Geometry check sheet. Reference: the model listing, model coordinates, mm. A direction names the side the tool comes from. Coordinates: 2 decimals unless noted, no trailing zeros. Write each loop counter-clockwise with the first axis right and the second up, starting at its lowest first coordinate (ties: lowest second). Pieces come first, ordered by that corner, then holes. Notation, with made-up numbers: (0.25, -7.75) -> (17.25, -7.75) arc R20 ccw to (17.25, 0.25) -> close; hole circle Ø11 at (-21, 83.5). An arc over 180 degrees is marked (long way). Answer in a Markdown table with one row per item. Add a question column.
1. Cross-section at B-B on z = 0. Record the cut outline in (x, y), and give its area (3 significant figures).
2. Cross-section at C-C on y = 182.5. Record the cut outline in (x, z).
3. Cross-section at A-A on x = 0. Record the cut outline in (y, z), and give its area (3 significant figures).
4. Set-up check for faces 4 (the cylindrical face through (3.69, 202.9, 51.92)), 5 (the flat face through (98.3, 20, 18.3)), 6 (the conical face through (-12.65, 102.63, -56.98)): record each of +Z, -Z, +X, -X, +Y, -Y from which the full face is reachable in a straight line by a thin tool's end or side.
5. Depth check by flat-ended pin: P1, Ø3, axis at x = -41.5, z = 73.5, coming from the -Y side; P2, Ø8, axis at y = 215, z = -56.5, coming from the +X side; P3, Ø12, axis at x = 25.5, z = -26, coming from the +Y side; P4, Ø12, axis at y = 36, z = 10, coming from the -X side. Enter the tip coordinate at first touch or a pass-through.
6. Scan lines: L1, parallel to Z at x = 0, y = 186; L2, parallel to Z at x = 0, y = 215; L3, parallel to Y at x = -83, z = -61. Record each from-to range of solid material in increasing order. Write a range as from..to.
7. Cross-section at D-D on y = 210. Record the cut outline in (x, z).
8. Mould release check, pull along Z, two halves, no side actions. Record for faces 1 (the cylindrical face through (-119.884, 9.86, 5.276)), 2 (the conical face through (-8.724, 245.243, -39.286)), 3 (the flat face through (-14, 250, 44)): pulls with the +Z half, pulls with the -Z half, needs draft (parallel to the pull), parting line crosses it, or undercut.
```python
from build123d import *

# Parameters (mm, degrees)
CHAMFER1_SIZE      = 5
SKETCH2_R          = 8
CUT_EXTRUDE1_DEPTH = 120


with BuildPart() as part:
    # Sketch1 → Revolve1 (revolve)
    with BuildSketch(Plane.XY):
        with BuildLine():
            Line((40, 250), (65, 250))
            Line((65, 250), (65, 170))
            ThreePointArc((65, 170), (60.268530098, 166.616537216), (61.940561127, 161.045277028))
            Line((61.940561127, 161.045277028), (90, 27.937311241))
            ThreePointArc((90, 27.937311241), (93.485226827, 22.233826953), (99.784953504, 20))
            Line((99.784953504, 20), (120, 20))
            Line((120, 20), (120, 0))
            Line((120, 0), (80, 0))
            Line((80, 0), (45, 166.032500638))
            ThreePointArc((45, 166.032500638), (43.215449857, 168.917888595), (40, 170))
            Line((40, 170), (40, 250))
        make_face()
    revolve(axis=Axis((0, 107.637867538, 0), (0, -1, 0)))

    # Chamfer1
    chamfer1_edges = [part.edges().sort_by_distance(p)[0] for p in [
        (-40, 250, 0),
    ]]
    chamfer(chamfer1_edges, length=CHAMFER1_SIZE)

    # Sketch2 → Cut-Extrude1 (cut)
    with BuildSketch(Plane.XY):
        with Locations((0, 210)):
            Circle(SKETCH2_R)
    extrude(amount=CUT_EXTRUDE1_DEPTH, mode=Mode.SUBTRACT)


solid = part.part
```
Results found:
| question | item | result |
|---|---|---|
| 1 | outline | (-120, 0) -> (-80, 0) -> (-45, 166.03) arc R5 cw to (-40, 170) -> (-40, 245) -> (-45, 250) -> (-65, 250) -> (-65, 170) arc R5 cw to (-61.94, 161.05) -> (-90, 27.94) arc R10 cw to (-99.78, 20) -> (-120, 20) -> close; (40, 170) arc R5 cw to (45, 166.03) -> (80, 0) -> (120, 0) -> (120, 20) -> (99.78, 20) arc R10 cw to (90, 27.94) -> (61.94, 161.05) arc R5 cw to (65, 170) -> (65, 250) -> (45, 250) -> (40, 245) -> close |
| 1 | area | 10,500 mm^2 |
| 2 | outline | circle Ø130 at (0, 0); hole circle Ø80 at (0, 0) |
| 3 | outline | (0, -120) -> (20, -120) -> (20, -99.78) arc R10 cw to (27.94, -90) -> (161.05, -61.94) arc R5 cw to (170, -65) -> (250, -65) -> (250, -45) -> (245, -40) -> (170, -40) arc R5 cw to (166.03, -45) -> (0, -80) -> close; (0, 80) -> (166.03, 45) arc R5 cw to (170, 40) -> (202, 40) -> (202, 65) -> (170, 65) arc R5 cw to (161.05, 61.94) -> (27.94, 90) arc R10 cw to (20, 99.78) -> (20, 120) -> (0, 120) -> close; (218, 40) -> (245, 40) -> (250, 45) -> (250, 65) -> (218, 65) -> close |
| 3 | area | 10,100 mm^2 |
| 4 | face 4 | +Z |
| 4 | face 5 | +Y |
| 4 | face 6 | -Y |
| 5 | P1 | stops at y = 0 |
| 5 | P2 | stops at x = 38.32 |
| 5 | P3 | stops at y = 247.42 |
| 5 | P4 | stops at x = -89.14 |
| 6 | L1 | z = -65..-40, 40..65 |
| 6 | L2 | z = -65..-40 |
| 6 | L3 | y = 0..20 |
| 7 | outline | (-8, 39.19) -> (-8, 64.51) arc R65 ccw (long way) to (8, 64.51) -> (8, 39.19) arc R40 cw (long way) to start |
| 8 | face 1 | parting line crosses it |
| 8 | face 2 | undercut |
| 8 | face 3 | needs draft |
